from build123d import *

# Parameters (mm, degrees)
CHAMFER1_SIZE      = 0.508
CHAMFER2_SIZE      = 1.524
CUT_EXTRUDE1_DEPTH = 49.26
FILLET1_R          = 0.762


with BuildPart() as part:
    # Sketch1 → Revolve1 (revolve)
    with BuildSketch(Plane.XY):
        with BuildLine():
            Line((0, 52.2986), (0, -30.2514))
            Line((0, -30.2514), (-15.875, -30.2514))
            Line((-15.875, -30.2514), (-15.875, -4.318))
            Line((-15.875, -4.318), (-13.6017, -4.318))
            Line((-13.6017, -4.318), (-13.6017, -1.27))
            ThreePointArc((-13.6017, -1.27), (-13.973674388, -0.371974388), (-14.8717, 0))
            Line((-14.8717, 0), (-21.5519, 0))
            Line((-21.5519, 0), (-21.5519, 18.0086))
            Line((-21.5519, 18.0086), (-15.0114, 18.0086))
            Line((-15.0114, 18.0086), (-15.0114, 34.036))
            ThreePointArc((-15.0114, 34.036), (-11.938, 38.6842), (-15.0114, 43.3324))
            Line((-15.0114, 43.3324), (-15.0114, 47.117))
            Line((-15.0114, 47.117), (-9.8298, 52.2986))
            Line((-9.8298, 52.2986), (0, 52.2986))
        make_face()
    revolve(axis=Axis((0, -30.2514, 0), (0, -1, 0)))

    # Chamfer1
    chamfer1_edges = [part.edges().sort_by_distance(p)[0] for p in [
        (21.5519, 18.0086, 0),
        (21.5519, 0, 0),
    ]]
    chamfer(chamfer1_edges, length=CHAMFER1_SIZE)

    # Chamfer2
    chamfer2_edges = [part.edges().sort_by_distance(p)[0] for p in [
        (15.875, -30.2514, 0),
    ]]
    chamfer(chamfer2_edges, length=CHAMFER2_SIZE)

    # Sketch2 → Cut-Extrude1 (cut, through all)
    with BuildSketch(Plane(origin=(0, 18.0086, 0), x_dir=(1, 0, 0), z_dir=(0, 1, 0))):
        with BuildLine():
            Line((-17.4244, 12.68363821), (-17.4244, -12.68363821))
            ThreePointArc((-17.4244, -12.68363821), (-21.5519, 0), (-17.4244, 12.68363821))
        make_face()
        with BuildLine():
            Line((17.4244, 12.68363821), (17.4244, -12.68363821))
            ThreePointArc((17.4244, -12.68363821), (21.5519, 0), (17.4244, 12.68363821))
        make_face()
    extrude(amount=-CUT_EXTRUDE1_DEPTH, mode=Mode.SUBTRACT)

    # Fillet1
    fillet1_edges = [part.edges().sort_by_distance(p)[0] for p in [
        (15.0114, 18.0086, 0),
    ]]
    fillet(fillet1_edges, radius=FILLET1_R)


solid = part.part
Geometry check sheet. Reference: the model listing, model coordinates, mm. A direction names the side the tool comes from. Give positions to 0.01 mm unless a question says otherwise; leave off trailing zeros. Order: outer loops, then holes, each group sorted by start corner. A loop starts at its lowest first (then second) coordinate and runs counter-clockwise, first axis right, second up. Notation, with made-up numbers: (-34.75, 88.5) - (-10.75, 88.5) arc R34 cw to (-10.75, 121.5) - close; hole circle Ø10 at (16.5, -1). An arc over 180 degrees is marked (long way). Answer as a JSON object with one key per item and string values.
(1) Depth check by flat-ended pin: pin 1 Ø5 at (x, y) = (-4, 1.5) entering from -Z; pin 2 Ø2 at (y, z) = (28.5, -8.5) entering from -X; pin 3 Ø1 at (x, y) = (-11, 22.5) entering from +Z. Enter the tip coordinate at first touch or a pass-through.
Report:
{"pin 1": "z = -21.5", "pin 2": "x = -13", "pin 3": "z = 10.73"}
(2) Cross-section at B-B (z = 0). Record the cut outline in (x, y) (3 decimals).
Report:
{"outline": "(-17.424, 0) - (-14.872, 0) arc R1.27 cw to (-13.602, -1.27) - (-13.602, -4.318) - (-15.875, -4.318) - (-15.875, -28.727) - (-14.351, -30.251) - (14.351, -30.251) - (15.875, -28.727) - (15.875, -4.318) - (13.602, -4.318) - (13.602, -1.27) arc R1.27 cw to (14.872, 0) - (17.424, 0) - (17.424, 18.009) - (15.773, 18.009) arc R0.762 cw to (15.011, 18.771) - (15.011, 34.036) arc R5.052 cw to (15.011, 43.332) - (15.011, 47.117) - (9.83, 52.299) - (-9.83, 52.299) - (-15.011, 47.117) - (-15.011, 43.332) arc R5.052 cw to (-15.011, 34.036) - (-15.011, 18.771) arc R0.762 cw to (-15.773, 18.009) - (-17.424, 18.009) - close"}
(3) Cross-section at C-C (y = -8.5). Record the cut outline in (x, z) (3 decimals), then the cut area to 3 significant figures.
Report:
{"outline": "circle Ø31.75 at (0, 0)", "area": "792 mm^2"}
(4) Tool access check on faces 4 (the cylindrical face through (-13, -3, -4)), 5 (the cylindrical face through (3.441, -16.352, 15.497)), 6 (the cylindrical face through (-14.318, 26.51, -4.509)). Record the directions out of +Z, -Z, +X, -X, +Y, -Y that give a thin tool (end or side, any length) a straight path to the whole face; none if there is none.
Report:
{"face 4": "none", "face 5": "-Y", "face 6": "+Y"}
(5) Cross-section at D-D (y = 41). Record the cut outline in (x, z).
Report:
{"outline": "circle Ø25 at (0, 0)"}
(6) Material ranges on line 1 (Y direction, x = -10.5, z = 10.5); line 2 (Y direction, x = 4.5, z = -16); line 3 (X direction, y = 24.5, z = -6), recorded low to high.
Report:
{"line 1": "-29.75 to -4.32, 0 to 34.11, 43.26 to 47.28", "line 2": "0 to 18.01", "line 3": "-13.76 to 13.76"}
(7) Draft check along Y on faces 1 (the flat face through (-12, -4.318, -7)), 2 (the conical face through (-0.289, 0.145, -21.187)), 3 (the conical face through (-0.29, 17.87, -21.18)). Enter one of: released by +Y, released by -Y, zero draft, split by the parting line, or undercut.
Report:
{"face 1": "undercut", "face 2": "released by -Y", "face 3": "released by +Y"}
